Geometry: final body of the model. Coordinates: model frame, mm. Face numbers are marked on the shaded views. A direction names the side the tool comes from. Round coordinates to 2 decimals unless told otherwise and drop trailing zeros. Loops run counter-clockwise (first coordinate to the right, second up) from the corner with the lowest first, then second, coordinate; pieces in that order, holes last. Notation, with made-up numbers: (49.5, 22.25) - (105.5, 22.25) arc R28 cw to (105.5, 41.25) - close; hole circle Ø1 at (57, -18). An arc over 180 degrees is marked (long way). Answer as CSV lines item,"result".
from build123d import *

# Parameters (mm, degrees)
SKETCH1_R           = 17
BOSS_EXTRUDE1_DEPTH = 3
SKETCH3_W           = 37.520369423
SKETCH3_H           = 53
SKETCH3_R           = 3.081115769
SKETCH3_W_2         = 8.431940609
SKETCH3_H_2         = 7.24288365
BOSS_EXTRUDE2_DEPTH = 3
SKETCH2_R           = 1.5
CUT_EXTRUDE1_DEPTH  = 3


with BuildPart() as part:
    # Sketch1 → Boss-Extrude1 (new body)
    with BuildSketch(Plane(origin=(0, 0, 0), x_dir=(1, 0, 0), z_dir=(0, 1, 0))):
        Polygon((-140.450145292, 142.201168563), (-100.450145292, 142.201168563), (-100.450145292, -7.798831437), (-140.450145292, -7.798831437), (-140.450145292, -284.717952364), (-190.450145292, -284.717952364), (-190.450145292, -7.798831437), (-250.450145292, -7.798831437), (-250.450145292, 142.201168563), (-200.450145292, 142.201168563), (-190.450145292, 142.201168563), (-190.450145292, 402.408103705), (-140.450145292, 402.408103705), align=None)
        with Locations(Location((-169.10841193, 373.953530137, 0), (0, 0, 270))):
            Circle(SKETCH1_R, mode=Mode.SUBTRACT)
        with Locations(Location((-169.10841193, -235.646469863, 0), (0, 0, 270))):
            Circle(SKETCH1_R, mode=Mode.SUBTRACT)
    extrude(amount=BOSS_EXTRUDE1_DEPTH)

    # Sketch3 → Boss-Extrude2 (add)
    with BuildSketch(Plane.ZY.offset(250.450145292)):
        with Locations((-70.700585856, 26.5)):
            Rectangle(SKETCH3_W, SKETCH3_H)
        with Locations((-71.485173946, 15.517365386)):
            Circle(SKETCH3_R, mode=Mode.SUBTRACT)
        with Locations((-70.350319411, 43.392750381)):
            Rectangle(SKETCH3_W_2, SKETCH3_H_2, mode=Mode.SUBTRACT)
    extrude(amount=BOSS_EXTRUDE2_DEPTH)

    # Sketch2 → Cut-Extrude1 (cut)
    with BuildSketch(Plane(origin=(0, 3, 0), x_dir=(1, 0, 0), z_dir=(0, 1, 0))):
        with Locations(Location((-236.200145292, 67.201168563, 0), (0, 0, 270))):
            Circle(SKETCH2_R)
        with Locations(Location((-172.579411925, 77.325298746, 0), (0, 0, 270))):
            Circle(SKETCH2_R)
        with Locations(Location((-132.001291312, 27.290192535, 0), (0, 0, 270))):
            Circle(SKETCH2_R)
        with Locations(Location((-155.043904065, -32.86904386, 0), (0, 0, 270))):
            Circle(SKETCH2_R)
        with Locations((-218.664637432, -42.993174043)):
            Circle(SKETCH2_R)
        with Locations((-259.242758045, 7.041932168)):
            Circle(SKETCH2_R)
    extrude(amount=-CUT_EXTRUDE1_DEPTH, mode=Mode.SUBTRACT)


solid = part.part
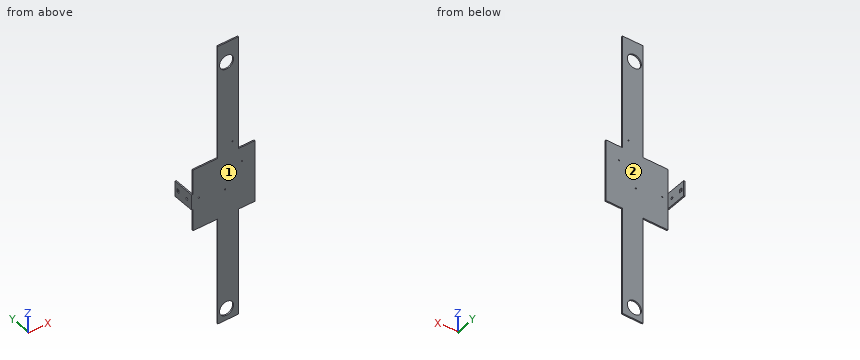
(1) Material intervals for line 1 along Y through (x, z) = (-175.5, 202); line 2 along X through (y, z) = (2.5, -347); line 3 along X through (y, z) = (36, -86), sorted ascending.
Findings below:
line 1,"0 to 3"
line 2,"-190.45 to -140.45"
line 3,"-253.45 to -250.45"
(2) Section C-C (z = -230). Output: boundary loops of the cut face in (x, y).
Findings below:
outline,"(-190.45, 0) - (-140.45, 0) - (-140.45, 3) - (-190.45, 3) - close"
(3) Pin query (flat end, axial travel): P1, Ø2.5, axis at y = 2, z = 96, coming from the +X side; P2, Ø3.5, axis at y = 2, z = -116, coming from the -X side; P3, Ø1.5, axis at x = -251.5, y = 30.5, coming from the +Z side. Return the tip coordinate at first contact, or that it passes through.
Findings below:
P1,"x = -140.45"
P2,"x = -250.45"
P3,"z = -51.94"
(4) Section A-A (x = -180). Output: boundary loops of the cut face in (y, z).
Findings below:
outline,"(0, -402.41) - (3, -402.41) - (3, -387.01) - (0, -387.01) - close; (0, -360.9) - (3, -360.9) - (3, 222.59) - (0, 222.59) - close; (0, 248.7) - (3, 248.7) - (3, 284.72) - (0, 284.72) - close"
(5) Access query for the marked faces 1 and 2. Directions: +Z, -Z, +X, -X, +Y, -Y. A direction counts if a zero-diameter tool reaches every point of the face in a straight line with its end or side. Return the directions, or none.
Findings below:
face 1,"+Z, -Z, +X, -X, -Y"
face 2,"+Z, -Z, +X, +Y"
(6) Section B-B (y = 33.5). Output: boundary loops of the cut face in (x, z), and give its area (3 significant figures).
Findings below:
outline,"(-253.45, -89.46) - (-250.45, -89.46) - (-250.45, -51.94) - (-253.45, -51.94) - close"
area,"113 mm2"
